Autodesk Inventor part; units mm, degrees
ref_plane "Start plane" through (0, 0, -8.9803) normal (0, 0, 1) x (1, 0, 0)
ref_plane "End plane" through (0, 0, 45.7894) normal (0, 0, 1) x (1, 0, 0)
ref_plane "Work Plane4" through (0, -70.5269, -76.3322) normal (0, 0.7071, -0.7071) x (1, 0, 0)
ref_plane "Start plane" through (0, 0, -8.9803) normal (0, 0, 1) x (1, 0, 0)
ref_plane "End plane" through (0, 0, 45.7894) normal (0, 0, 1) x (1, 0, 0)
sketch "Sketch" plane through (0, 0, 0) normal (0, 0, 1) x (1, 0, 0)
  line L0 (12.7, -3.175) -> (-12.7, -3.175)
  line L1 (-12.7, -3.175) -> (-12.7, 3.175)
  line L2 (-12.7, 3.175) -> (12.7, 3.175)
  line L3 (12.7, 3.175) -> (12.7, -3.175)
  line L4 (-6, 0) -> (8, 0) construction
  line L5 (0, -30) -> (0, 40) construction
  line L6 (0, 54) -> (0, -44) construction
  line L7 (-17.78, 0) -> (17.78, 0) construction
  dimension "d0" = 6.35
  dimension "d1" = 25.4
  dimension "d4" = 12.7
  dimension "d5" = 3.175
extrude "Body" add sketch "Sketch" along normal up to surface (54.7697 mm away) from surface at -8.9803
sketch "Sketch3" plane through (0, 0, 0) normal (0, 0, 1) x (1, 0, 0)
  line L0 (0, 0) -> (10, 0)
ref_plane "Work Plane3" through (0, 0, 0) normal (0, -1, 0) x (1, 0, 0)
sketch "Sketch4" plane through (0, 0, 0) normal (0, -1, 0) x (1, 0, 0)
  line L0 (-2, -8.9803) -> (12, -8.9803)
  line L1 (-2, 45.7894) -> (12, 45.7894)
  dimension "d9" = 54.7697
ref_plane "Work Plane4" through (0, -70.5269, -76.3322) normal (0, 0.7071, -0.7071) x (1, 0, 0)
split "Split1" plane through (0, -70.5269, -76.3322) removes the side toward (0, 0.7071, -0.7071)
ref_plane "Work Plane5" through (0, 5.3513, 37.2631) normal (0, 0.7071, 0.7071) x (1, 0, 0)
split "Split2" plane through (0, 5.3513, 37.2631) removes the side toward (0, 0.7071, 0.7071)
equation "\"d0\" = G_W"
equation "\"d1\" = G_H"
equation "\"d4\" = 0.5 * d1"
equation "\"d5\" = 0.5 * d0"
equation "\"d2\" = G_L"
equation "\"G_W\" = 6.35"
equation "\"G_H\" = 25.4"
equation "\"G_L\" = d9"
equation "\"G_OFFSET_START\" = 8.98026"
equation "\"G_OFFSET_END\" = 17.05259"
equation "\"d6\" = -G_OFFSET_START"
equation "\"d7\" = G_OFFSET_END + B_L"
equation "\"B_L\" = 28.73682"
properties part number "AISC - 1/4x1 - 2.156" material "Steel, Mild"
Geometry check sheet. Reference: the model listing, model coordinates, mm. Coordinates: 2 decimals unless noted, no trailing zeros. Write each loop counter-clockwise with the first axis right and the second up, starting at its lowest first coordinate (ties: lowest second). Pieces come first, ordered by that corner, then holes. Notation, with made-up numbers: (-28, -26.5) -> (-24, -26.5) arc R34 ccw to (-24, 10.5) -> close; hole circle Ø6 at (45, -11.75). An arc over 180 degrees is marked (long way). One line per question, with ' | ' between items.
1. Depth check by flat-ended pin: pin 1 Ø1 at (x, y) = (-7.5, 2.5) entering from +Z. Enter the tip coordinate at first touch or a pass-through.
Answers:
pin 1: stops at z = 40.61
2. Cross-section at B-B on y = -0.25. Record the cut outline in (x, z), and give its area (3 significant figures).
Answers:
outline: (-12.7, -6.06) -> (12.7, -6.06) -> (12.7, 42.86) -> (-12.7, 42.86) -> close | area: 1,240 mm²
3. Cross-section at A-A on x = -4. Record the cut outline in (y, z) (3 decimals).
Answers:
outline: (-3.175, -8.98) -> (3.175, -2.63) -> (3.175, 39.439) -> (-3.175, 45.789) -> close
4. Thickness scan on probe 1 along Z at (x, y) = (-9.5, 0.5); probe 2 along Z at (x, y) = (7.5, -1.75); probe 3 along Y at (x, z) = (11.75, -3.5) (3 decimals). Record the ranges inside material, lowest first. Write a range as from..to.
Answers:
probe 1: z = -5.31..42.11 | probe 2: z = -7.56..44.36 | probe 3: y = -3.175..2.305
